Geometry: see drawing. Coordinates: mm, zero at the bounding-box minimum. A direction names the side the tool comes from. Give positions to 0.01 mm unless a question says otherwise; leave off trailing zeros. Order: outer loops, then holes, each group sorted by start corner. A loop starts at its lowest first (then second) coordinate and runs counter-clockwise, first axis right, second up. Notation, with made-up numbers: (32, 83) - (39, 83) arc R29 cw to (39, 117) - close; hole circle Ø7 at (81.25, -18.75). An arc over 180 degrees is marked (long way). Write item = value, one per line. Start each with the question number.
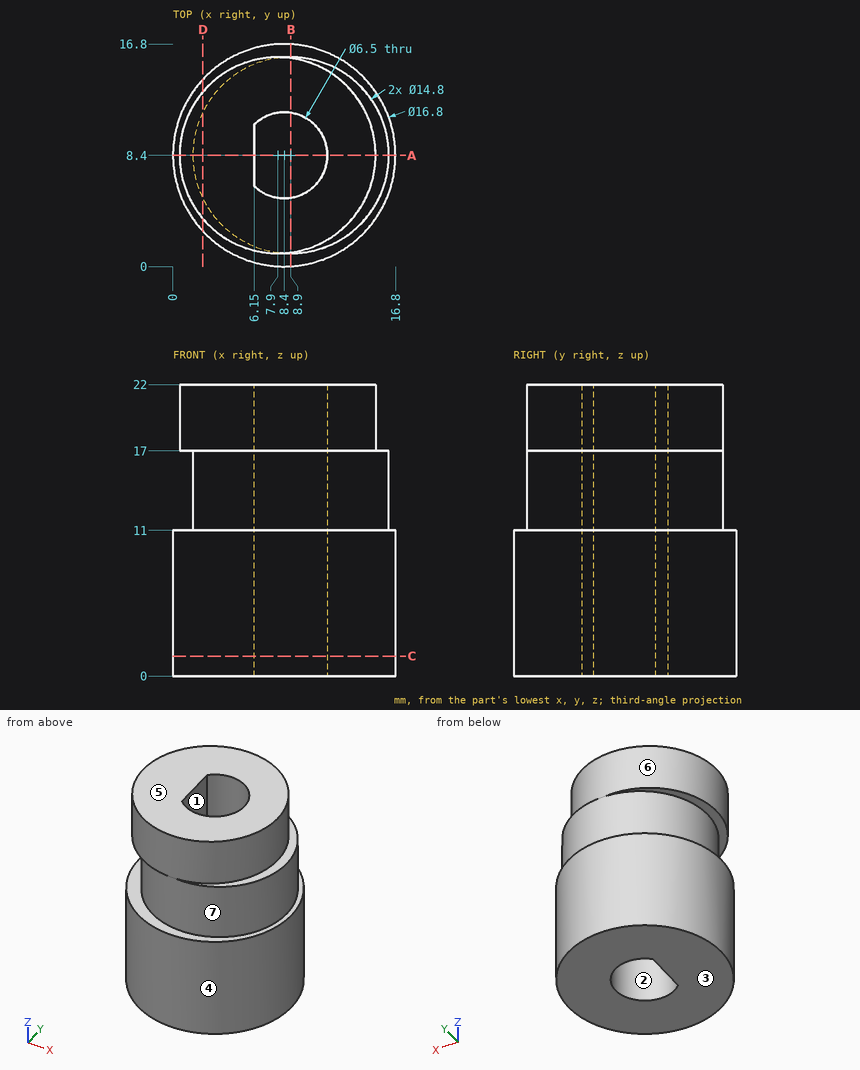
Q1. Pull-direction query (Y, two-part tool) for the marked faces 1, 2, 3 and 4; classes: +Y half, -Y half, draft (parallel to the pull), parting line (faces both ways), or undercut.
Q2. Section C-C, the plane z = 1.5. Return the cut outline in (x, y).
Q3. Section A-A, the plane y = 8.4. Return the cut outline in (x, z), then the cut area to 3 significant figures.
Q4. Material intervals for line 1 along Y through (x, z) = (8.4, 5.75); line 2 along X through (y, z) = (8.4, 15.5); line 3 along Z through (x, y) = (15.25, 13), sorted ascending. Write a range as from..to.
Q5. Contact query for flat-ended pins moving along their axis: pin 1 (1 mm diameter, centred on y = 13.5, z = 13.5, fed in from +X); pin 2 (8 mm diameter, centred on x = 4.5, z = 18, fed in from -Y); pin 3 (3 mm diameter, centred on y = 6.5, z = 13.5, fed in from -X); pin 4 (4 mm diameter, centred on x = 8.4, y = 8.4, fed in from +Z). Output: stop coordinate, or through.
Q6. Section B-B, the plane x = 8.9. Return the cut outline in (y, z).
Q7. Section D-D, the plane x = 2.25. Return the cut outline in (y, z), then the cut area to 3 significant figures.
Q8. Set-up query: the marked faces 5, 6 and 7. Return all of +Z, -Z, +X, -X, +Y, -Y with unobstructed straight access to the full face (end or side cutting, diameter ignored); none if empty.
The answers:
q1.face_1 = undercut
q1.face_2 = undercut
q1.face_3 = draft
q1.face_4 = parting line
q2.outline = circle Ø16.8 at (8.4, 8.4); hole (6.15, 6.05) arc R3.25 ccw (long way) to (6.15, 10.75) - close
q3.outline = (0, 0) - (6.15, 0) - (6.15, 22) - (0.5, 22) - (0.5, 17) - (1.5, 17) - (1.5, 11) - (0, 11) - close; (11.65, 0) - (16.8, 0) - (16.8, 11) - (16.3, 11) - (16.3, 17) - (15.3, 17) - (15.3, 22) - (11.65, 22) - close
q3.area = 227 mm²
q4.line_1 = 0..5.15, 11.65..16.8
q4.line_2 = 1.5..6.15, 11.65..16.3
q4.line_3 = 0..11
q5.pin_1 = 14.7
q5.pin_2 = 1
q5.pin_3 = 1.51
q5.pin_4 = through
q6.outline = (0.01, 0) - (5.19, 0) - (5.19, 22) - (1.07, 22) - (1.07, 17) - (1, 17) - (1, 11) - (0.01, 11) - close; (11.61, 0) - (16.79, 0) - (16.79, 11) - (15.8, 11) - (15.8, 17) - (15.73, 17) - (15.73, 22) - (11.61, 22) - close
q7.outline = (2.68, 0) - (14.12, 0) - (14.12, 11) - (11.65, 11) - (11.65, 17) - (13.18, 17) - (13.18, 22) - (3.62, 22) - (3.62, 17) - (5.15, 17) - (5.15, 11) - (2.68, 11) - close
q7.area = 213 mm²
q8.face_5 = +Z, +X, -X, +Y, -Y
q8.face_6 = +Z
q8.face_7 = none
